```python
from build123d import *

# Parameters (mm, degrees)
F0_R     = 2.5527
F0_R_2   = 1.9939
F0_R_3   = 3.5687
F1_DEPTH = 5.9944
F2_W     = 19.9898
F2_H     = 24.003
F2_R     = 1.9939
F3_DEPTH = 6.985
F4_R     = 1.5494
F5_DEPTH = 11.9888
F7_D     = 2.9972


with BuildPart() as f1:
    # F0 (on Front) → F1 (new body)
    with BuildSketch(Plane.XZ):
        with BuildLine():
            ThreePointArc((40.2971, 13.0048), (37.9536613563, 18.6623613563), (32.2961, 21.0058))
            Line((32.2961, 21.0058), (-32.2961, 21.0058))
            ThreePointArc((-32.2961, 21.0058), (-37.9536613563, 18.6623613563), (-40.2971, 13.0048))
            Line((-40.2971, 13.0048), (-40.2971, -13.0048))
            ThreePointArc((-40.2971, -13.0048), (-37.9536613563, -18.6623613563), (-32.2961, -21.0058))
            Line((-32.2961, -21.0058), (32.2961, -21.0058))
            ThreePointArc((32.2961, -21.0058), (37.9536613563, -18.6623613563), (40.2971, -13.0048))
            Line((40.2971, -13.0048), (40.2971, 13.0048))
        make_face()
        with Locations((-26.0731, -13.0048)):
            Circle(F0_R, mode=Mode.SUBTRACT)
        with Locations((2.438410781, -15.0241)):
            Circle(F0_R_2, mode=Mode.SUBTRACT)
        with BuildLine():
            Line((13.1191, -16.9164), (9.9187, -16.9164))
            ThreePointArc((9.9187, -16.9164), (8.0137, -15.0114), (9.9187, -13.1064))
            Line((9.9187, -13.1064), (13.1191, -13.1064))
            ThreePointArc((13.1191, -13.1064), (15.0241, -15.0114), (13.1191, -16.9164))
        make_face(mode=Mode.SUBTRACT)
        with Locations((2.438410781, -3.0099)):
            Circle(F0_R_2, mode=Mode.SUBTRACT)
        with BuildLine():
            Line((13.1191, -4.9022), (9.9187, -4.9022))
            ThreePointArc((9.9187, -4.9022), (8.0137, -2.9972), (9.9187, -1.0922))
            Line((9.9187, -1.0922), (13.1191, -1.0922))
            ThreePointArc((13.1191, -1.0922), (15.0241, -2.9972), (13.1191, -4.9022))
        make_face(mode=Mode.SUBTRACT)
        with Locations((-26.0731, 13.0048)):
            Circle(F0_R, mode=Mode.SUBTRACT)
        with Locations((25.8064, 0)):
            Circle(F0_R_3, mode=Mode.SUBTRACT)
    extrude(amount=F1_DEPTH)

    # F2 (on Front) → F3 (join)
    with BuildSketch(Plane.XZ):
        with Locations((6.985, -9.0043)):
            Rectangle(F2_W, F2_H)
        with Locations((2.438410781, -15.0241)):
            Circle(F2_R, mode=Mode.SUBTRACT)
        with BuildLine():
            Line((13.1191, -16.9164), (9.9187, -16.9164))
            ThreePointArc((9.9187, -16.9164), (8.0137, -15.0114), (9.9187, -13.1064))
            Line((9.9187, -13.1064), (13.1191, -13.1064))
            ThreePointArc((13.1191, -13.1064), (15.0241, -15.0114), (13.1191, -16.9164))
        make_face(mode=Mode.SUBTRACT)
        with Locations((2.438410781, -3.0099)):
            Circle(F2_R, mode=Mode.SUBTRACT)
        with BuildLine():
            Line((13.1191, -4.9022), (9.9187, -4.9022))
            ThreePointArc((9.9187, -4.9022), (8.0137, -2.9972), (9.9187, -1.0922))
            Line((9.9187, -1.0922), (13.1191, -1.0922))
            ThreePointArc((13.1191, -1.0922), (15.0241, -2.9972), (13.1191, -4.9022))
        make_face(mode=Mode.SUBTRACT)
    extrude(amount=F3_DEPTH)

    # F4 (on face) → F5 (join)
    with BuildSketch(Plane.XY.offset(21.0058)):
        Polygon((14.1859, -5.9944), (-14.1859, -5.9944), (-14.1859, -15.494), (-7.6835, -21.9964), (0.1905, -21.9964), (0.1905, -16.002), (12.6873, -16.002), (14.1859, -14.5034), align=None)
        with Locations((-6.3627, -18.9992)):
            Circle(F4_R, mode=Mode.SUBTRACT)
    extrude(amount=-F5_DEPTH)

    # F7 (through all)
    with Locations(Plane.YZ.offset(14.1859)):
        with Locations((-11.9888, 15.0114)):
            Hole(F7_D / 2)


solid = f1.part
```
Verification items for the finished model (mm, model axes). A direction names the side the tool comes from. Coordinates: 2 decimals unless noted, no trailing zeros. Order: outer loops, then holes, each group sorted by start corner. A loop starts at its lowest first (then second) coordinate and runs counter-clockwise, first axis right, second up. Notation, with made-up numbers: (-22.5, 24.5) -> (23.5, 24.5) arc R14 cw to (23.5, 40.5) -> close; hole circle Ø5 at (10, 63). An arc over 180 degrees is marked (long way). Put each result on its own line as item: value. Start each with the question number.
1) Go/stop test with flat-tipped pins: pin 1 (3 mm diameter, centred on y = -11.5, z = 13.5, fed in from -X); pin 2 (6 mm diameter, centred on x = -26, z = 10, fed in from -Y); pin 3 (16 mm diameter, centred on x = 3.5, z = -7.5, fed in from -Y) (3 decimals); pin 4 (1 mm diameter, centred on x = 8, y = -17, fed in from -Z). Record where each tip stops, or that it passes through.
2) Cross-section at A-A (z = 0). Enter the section's corners in (x, y) (3 decimals).
3) Material ranges on L1, parallel to Y at x = 10.5, z = 15; L2, parallel to Z at x = 1, y = -3.25; L3, parallel to Y at x = 18, z = 6, recorded low to high.
4) Tool access check on faces 5 (the flat face through (0, -6, 21.006)), 6 (the flat face through (-1, 0, 0)), 7 (the flat face through (0.19, -19, 15)), 8 (the flat face through (-14.186, -10, 15)), 9 (the cylindrical face through (8.014, -3.444, -15.053)). Record the directions out of +Z, -Z, +X, -X, +Y, -Y that give a thin tool (end or side, any length) a straight path to the whole face; none if there is none.
5) Cross-section at C-C (x = -4). Enter the section's corners in (y, z), plus the area to 3 significant figures.
6) Cross-section at B-B (y = -19.75). Enter the section's corners in (x, z), plus the area to 3 significant figures.
7) Cross-section at D-D (z = 8). Enter the section's corners in (x, y), plus the area to 3 significant figures.
8) Release check for a two-part mould opening along Z. For faces 1 (the cylindrical face through (-37.891, -2.955, 18.724)), 2 (the flat face through (-4, -21.996, 15)), 3 (the cylindrical face through (8.014, -3.444, -3.039)), 4 (the cylindrical face through (-38.016, -2.955, -18.6)) record: pulls with the +Z half, pulls with the -Z half, needs draft (parallel to the pull), parting line crosses it, or undercut.
Geometry check:
1. pin 1: stops at x = -14.19
1. pin 2: stops at y = -5.99
1. pin 3: stops at y = -6.985
1. pin 4: passes through
2. outline: (-40.297, -5.994) -> (-3.01, -5.994) -> (-3.01, -6.985) -> (16.98, -6.985) -> (16.98, -5.994) -> (22.238, -5.994) -> (22.238, 0) -> (-40.297, 0) -> close; (29.375, -5.994) -> (40.297, -5.994) -> (40.297, 0) -> (29.375, 0) -> close
3. L1: y = -16 to -13.49, -10.49 to 0
3. L2: z = -21.01 to -16.4, -13.64 to -4.39, -1.63 to 21.01
3. L3: y = -5.99 to 0
4. face 5: +Z, +X, -X, +Y, -Y
4. face 6: +Z, -Z, +X, -X, +Y
4. face 7: +Z, -Z, +X, -Y
4. face 8: +Z, -Z, -X, -Y
4. face 9: +Y, -Y
5. outline: (-22, 9.02) -> (-5.99, 9.02) -> (-5.99, -21.01) -> (0, -21.01) -> (0, 21.01) -> (-22, 21.01) -> close; hole circle Ø3 at (-11.99, 15.01)
5. area: 437 mm^2
6. outline: (-9.93, 9.02) -> (-7.72, 9.02) -> (-7.72, 21.01) -> (-9.93, 21.01) -> close; (-5.01, 9.02) -> (0.19, 9.02) -> (0.19, 21.01) -> (-5.01, 21.01) -> close
6. area: 88.8 mm^2
7. outline: (-40.3, -5.99) -> (40.3, -5.99) -> (40.3, 0) -> (-40.3, 0) -> close
7. area: 483 mm^2
8. face 1: pulls with the +Z half
8. face 2: needs draft
8. face 3: undercut
8. face 4: pulls with the -Z half
